from build123d import *

# Parameters (mm, degrees)
SKETCH1_R           = 2.7051
BOSS_EXTRUDE1_DEPTH = 1.1
SKETCH2_R           = 2.7051
SKETCH2_R_2         = 1.9431
BOSS_EXTRUDE2_DEPTH = 2.25
SKETCH3_R           = 0.930000045
CUT_EXTRUDE1_DEPTH  = 14.668625754
CUT_EXTRUDE2_REACH  = 15.669
SKETCH4_R           = 0.575


with BuildPart() as part:
    # Sketch1 → Boss-Extrude1 (new body)
    with BuildSketch(Plane(origin=(0, 0, 0), x_dir=(1, 0, 0), z_dir=(0, 1, 0))):
        with BuildLine():
            Line((-2.185682545, 1.59385), (-11.61415, 1.59385))
            ThreePointArc((-11.61415, 1.59385), (-13.208, 0), (-11.61415, -1.59385))
            Line((-11.61415, -1.59385), (-2.185682545, -1.59385))
            ThreePointArc((-2.185682545, -1.59385), (-2.7051, 0), (-2.185682545, 1.59385))
        make_face()
        Circle(SKETCH1_R)
    extrude(amount=BOSS_EXTRUDE1_DEPTH)

    # Sketch2 → Boss-Extrude2 (add)
    with BuildSketch(Plane(origin=(0, 1.1, 0), x_dir=(1, 0, 0), z_dir=(0, 1, 0))):
        with Locations(Location((0, 0, 0), (0, 0, 143.899608526))):
            Circle(SKETCH2_R)
        with Locations(Location((0, 0, 0), (0, 0, 270))):
            Circle(SKETCH2_R_2, mode=Mode.SUBTRACT)
    extrude(amount=BOSS_EXTRUDE2_DEPTH)

    # Sketch3 → Cut-Extrude1 (cut, through all)
    with BuildSketch(Plane(origin=(0, 1.1, 0), x_dir=(1, 0, 0), z_dir=(0, 1, 0))):
        with Locations(Location((0, 0, 0), (0, 0, 270))):
            Circle(SKETCH3_R)
    extrude(amount=-CUT_EXTRUDE1_DEPTH, mode=Mode.SUBTRACT)

    # Sketch4 → Cut-Extrude2 (cut, up to next)
    with BuildSketch(Plane(origin=(0, 1.1, 0), x_dir=(1, 0, 0), z_dir=(0, 1, 0)), mode=Mode.PRIVATE) as cut_extrude2_sk1:
        with Locations(Location((-11.61415, 0, 0), (0, 0, 270))):
            Circle(SKETCH4_R)
    cut_extrude2_tool1 = extrude(cut_extrude2_sk1.sketch, amount=-CUT_EXTRUDE2_REACH, mode=Mode.PRIVATE) & part.part
    # Sketch4 → Cut-Extrude2 (cut, up to next)
    with BuildSketch(Plane(origin=(0, 1.1, 0), x_dir=(1, 0, 0), z_dir=(0, 1, 0)), mode=Mode.PRIVATE) as cut_extrude2_sk2:
        with Locations(Location((-9.01415, 0, 0), (0, 0, 270))):
            Circle(SKETCH4_R)
    cut_extrude2_tool2 = extrude(cut_extrude2_sk2.sketch, amount=-CUT_EXTRUDE2_REACH, mode=Mode.PRIVATE) & part.part
    # Sketch4 → Cut-Extrude2 (cut, up to next)
    with BuildSketch(Plane(origin=(0, 1.1, 0), x_dir=(1, 0, 0), z_dir=(0, 1, 0)), mode=Mode.PRIVATE) as cut_extrude2_sk3:
        with Locations(Location((-6.41415, 0, 0), (0, 0, 270))):
            Circle(SKETCH4_R)
    cut_extrude2_tool3 = extrude(cut_extrude2_sk3.sketch, amount=-CUT_EXTRUDE2_REACH, mode=Mode.PRIVATE) & part.part
    add(cut_extrude2_tool1.solids().sort_by_distance((-11.61415, 1.1, 0))[0], mode=Mode.SUBTRACT)
    add(cut_extrude2_tool2.solids().sort_by_distance((-9.01415, 1.1, 0))[0], mode=Mode.SUBTRACT)
    add(cut_extrude2_tool3.solids().sort_by_distance((-6.41415, 1.1, 0))[0], mode=Mode.SUBTRACT)


solid = part.part
Design review of the part built by this model. Coordinates are the model's own, in mm. A direction names the side the tool comes from. Give positions to 0.01 mm unless a question says otherwise; leave off trailing zeros. Loops run counter-clockwise (first coordinate to the right, second up) from the corner with the lowest first, then second, coordinate; pieces in that order, holes last. Notation, with made-up numbers: M -35.75,7.25 L 18.25,7.25 A19 cw 18.25,31.25 Z; hole C -36,24 d7. An arc over 180 degrees is marked long. Answer as a JSON object with one key per item and string values.
Item 1: Machinability: for faces 4 (the face through (-6.8, 0.5, -1.594)), 5 (the face through (1.927, 2.209, -0.253)), 6 (the face through (-5, 0, 0)), 7 (the face through (-7, 0.5, 1.594)), which of the approach directions +Z, -Z, +X, -X, +Y, -Y give a long, thin tool a straight path to every point of the face, cutting with its end or side? Answer none if there is none.
Output values:
{"face 4": "-Z, -X, +Y, -Y", "face 5": "+Y", "face 6": "+Z, -Z, +X, -X, -Y", "face 7": "+Z, -X, +Y, -Y"}
Item 2: We need section A-A (z = 0). State the section outline as (x, y) points.
Output values:
{"outline": "M -13.21,0 L -12.19,0 L -12.19,1.1 L -13.21,1.1 Z; M -11.04,0 L -9.59,0 L -9.59,1.1 L -11.04,1.1 Z; M -8.44,0 L -6.99,0 L -6.99,1.1 L -8.44,1.1 Z; M -5.84,0 L -0.93,0 L -0.93,1.1 L -1.94,1.1 L -1.94,3.35 L -2.71,3.35 L -2.71,1.1 L -5.84,1.1 Z; M 0.93,0 L 2.71,0 L 2.71,3.35 L 1.94,3.35 L 1.94,1.1 L 0.93,1.1 Z"}
Item 3: Mouldability with a two-part tool opening along X and no side actions: class faces 1 (the face through (-13.208, 0.542, -0.035)), 2 (the face through (-12.175, 0.558, -0.125)), 3 (the face through (-8, 1.1, 0)) as pulls with the +X half, pulls with the -X half, needs draft (parallel to the pull), parting line crosses it, or undercut.
Output values:
{"face 1": "pulls with the -X half", "face 2": "undercut", "face 3": "needs draft"}
Item 4: We need section D-D (y = 1.85). State the section outline as (x, z) points.
Output values:
{"outline": "C 0,0 d5.41; hole C 0,0 d3.89"}
Item 5: For P1, Ø0.6, axis at x = -7, y = 0.5, coming from the -Z side; P2, Ø1, axis at x = -5.5, z = 0, coming from the +Y side; P3, Ø1.5, axis at y = 2.5, z = 0, coming from the -X side; P4, Ø1.8, axis at x = -9.01, z = 0, coming from the -Y side, all flat-tipped, find the tip position at first contact; note any pin that passes through.
Output values:
{"P1": "stops at z = -1.59", "P2": "stops at y = 1.1", "P3": "stops at x = -2.71", "P4": "stops at y = 0"}
Item 6: We need section B-B (x = 0). State the section outline as (y, z) points, and give its area (3 significant figures).
Output values:
{"outline": "M 0,-2.71 L 3.35,-2.71 L 3.35,-1.94 L 1.1,-1.94 L 1.1,-0.93 L 0,-0.93 Z; M 0,0.93 L 1.1,0.93 L 1.1,1.94 L 3.35,1.94 L 3.35,2.71 L 0,2.71 Z", "area": "7.33 mm2"}
Item 7: We need section C-C (y = 0.5). State the section outline as (x, z) points (3 decimals).
Output values:
{"outline": "M -11.614,-1.594 L -2.186,-1.594 A2.705 ccw long -2.186,1.594 L -11.614,1.594 A1.594 ccw Z; hole C -11.614,0 d1.15; hole C -9.014,0 d1.15; hole C -6.414,0 d1.15; hole C 0,0 d1.86"}
Item 8: Wall thickness on line 1 along X through (y, z) = (0.5, 0); line 2 along Y through (x, z) = (-8.75, 0.6); line 3 along X through (y, z) = (2.5, -0.2): over which ranges is each line inside the solid? List them lowest first.
Output values:
{"line 1": "x = -13.21 to -12.19, -11.04 to -9.59, -8.44 to -6.99, -5.84 to -0.93, 0.93 to 2.71", "line 2": "y = 0 to 1.1", "line 3": "x = -2.7 to -1.93, 1.93 to 2.7"}
